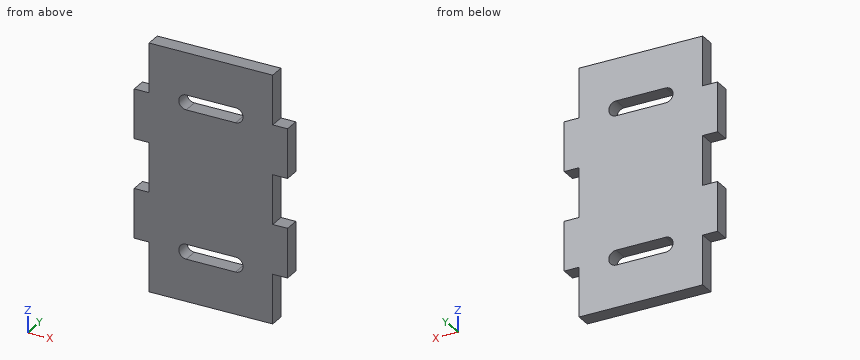
from build123d import *

# Parameters (mm, degrees)
SKETCH1_W           = 25
SKETCH1_H           = 50
BOSS_EXTRUDE1_DEPTH = 3
SKETCH2_W           = 3
SKETCH2_H           = 10
BOSS_EXTRUDE2_DEPTH = 3


with BuildPart() as part:
    # Sketch1 → Boss-Extrude1 (new body)
    with BuildSketch(Plane(origin=(0, 0, 0), x_dir=(1, 0, 0), z_dir=(0, 1, 0))):
        Rectangle(SKETCH1_W, SKETCH1_H)
        with BuildLine():
            Line((-5, 16.5), (5, 16.5))
            ThreePointArc((5, 16.5), (6.5, 15), (5, 13.5))
            Line((5, 13.5), (-5, 13.5))
            ThreePointArc((-5, 13.5), (-6.5, 15), (-5, 16.5))
        make_face(mode=Mode.SUBTRACT)
        with BuildLine():
            Line((-5, -16.5), (5, -16.5))
            ThreePointArc((5, -16.5), (6.5, -15), (5, -13.5))
            Line((5, -13.5), (-5, -13.5))
            ThreePointArc((-5, -13.5), (-6.5, -15), (-5, -16.5))
        make_face(mode=Mode.SUBTRACT)
    extrude(amount=BOSS_EXTRUDE1_DEPTH)

    # Sketch2 → Boss-Extrude2 (add)
    with BuildSketch(Plane(origin=(0, 3, 0), x_dir=(1, 0, 0), z_dir=(0, 1, 0))):
        with Locations((14, 10)):
            Rectangle(SKETCH2_W, SKETCH2_H)
        with Locations((14, -10)):
            Rectangle(SKETCH2_W, SKETCH2_H)
        with Locations((-14, -10)):
            Rectangle(SKETCH2_W, SKETCH2_H)
        with Locations((-14, 10)):
            Rectangle(SKETCH2_W, SKETCH2_H)
    extrude(amount=-BOSS_EXTRUDE2_DEPTH)


solid = part.part
Design review of the part built by this model. Coordinates are the model's own, in mm. Give positions to 0.01 mm unless a question says otherwise; leave off trailing zeros. Write each loop counter-clockwise with the first axis right and the second up, starting at its lowest first coordinate (ties: lowest second). Pieces come first, ordered by that corner, then holes. Notation, with made-up numbers: M -14.75,74.25 L 18.25,74.25 A21 cw 18.25,81.25 Z; hole C 59.5,-11 d8. An arc over 180 degrees is marked long. Return JSON: item names as keys, results as strings. Group by question number.
Item 1: Take a section at B-B (x = 1). Give the boundary of the cut face in (y, z), plus the area to 3 significant figures.
Item 2: Take a section at C-C (z = 22). Give the boundary of the cut face in (x, y).
Item 3: Wall thickness on line 1 along Z through (x, y) = (2.5, 2.2); line 2 along Z through (x, y) = (13.5, 0.4); line 3 along Z through (x, y) = (6, 0.75): over which ranges is each line inside the solid? List them lowest first.
Item 4: Take a section at A-A (y = 2.25). Give the boundary of the cut face in (x, z), plus the area to 3 significant figures.
Item 5: Clearance check with flat-ended pins moving along their axes: pin 1 Ø1.5 at (y, z) = (2, 20) entering from -X; pin 2 Ø0.9 at (x, y) = (-14, 1) entering from +Z; pin 3 Ø1.5 at (y, z) = (1.5, 20.5) entering from +X. State where each tip first meets the part, or that it passes through.
Return value:
{
 "1": {"outline": "M 0,-25 L 3,-25 L 3,-16.5 L 0,-16.5 Z; M 0,-13.5 L 3,-13.5 L 3,13.5 L 0,13.5 Z; M 0,16.5 L 3,16.5 L 3,25 L 0,25 Z", "area": "132 mm2"},
 "2": {"outline": "M -12.5,0 L 12.5,0 L 12.5,3 L -12.5,3 Z"},
 "3": {"line 1": "z = -25 to -16.5, -13.5 to 13.5, 16.5 to 25", "line 2": "z = -15 to -5, 5 to 15", "line 3": "z = -25 to -16.12, -13.88 to 13.88, 16.12 to 25"},
 "4": {"outline": "M -15.5,-15 L -12.5,-15 L -12.5,-25 L 12.5,-25 L 12.5,-15 L 15.5,-15 L 15.5,-5 L 12.5,-5 L 12.5,5 L 15.5,5 L 15.5,15 L 12.5,15 L 12.5,25 L -12.5,25 L -12.5,15 L -15.5,15 L -15.5,5 L -12.5,5 L -12.5,-5 L -15.5,-5 Z; hole M -5,-16.5 L 5,-16.5 A1.5 ccw 5,-13.5 L -5,-13.5 A1.5 ccw Z; hole M -5,13.5 L 5,13.5 A1.5 ccw 5,16.5 L -5,16.5 A1.5 ccw Z", "area": "1,300 mm2"},
 "5": {"pin 1": "stops at x = -12.5", "pin 2": "stops at z = 15", "pin 3": "stops at x = 12.5"}
}
